The model under review builds one solid part; all positions refer to its coordinate system, in mm. A direction names the side the tool comes from. Coordinates: 2 decimals unless noted, no trailing zeros. Write each loop counter-clockwise with the first axis right and the second up, starting at its lowest first coordinate (ties: lowest second). Pieces come first, ordered by that corner, then holes. Notation, with made-up numbers: (7.5, -7) - (37.5, -7) arc R25 cw to (37.5, 21) - close; hole circle Ø9 at (-25, 58). An arc over 180 degrees is marked (long way). Put each result on its own line as item: value.
from build123d import *

# Parameters (mm, degrees)
SKETCH_W        = 40
SKETCH_H        = 40
SKETCH_R        = 6
SKETCH_R_2      = 1.75
PAD_DEPTH       = 8
SKETCH001_R     = 9.7
POCKET_DEPTH    = 6
SKETCH002_W     = 42
SKETCH002_H     = 42
SKETCH002_R     = 15
POCKET001_DEPTH = 5
FILLET_R        = 3
FILLET001_R     = 3


with BuildPart() as part:
    # Sketch → Pad (new body)
    with BuildSketch(Plane.XY):
        Rectangle(SKETCH_W, SKETCH_H)
        Circle(SKETCH_R, mode=Mode.SUBTRACT)
        with Locations((15.6, 15.6)):
            Circle(SKETCH_R_2, mode=Mode.SUBTRACT)
        with Locations((15.6, -15.6)):
            Circle(SKETCH_R_2, mode=Mode.SUBTRACT)
        with Locations((-15.6, -15.6)):
            Circle(SKETCH_R_2, mode=Mode.SUBTRACT)
        with Locations((-15.6, 15.6)):
            Circle(SKETCH_R_2, mode=Mode.SUBTRACT)
    extrude(amount=PAD_DEPTH)

    # Sketch001 → Pocket (cut)
    with BuildSketch(Plane.XY.offset(8)):
        Circle(SKETCH001_R)
    extrude(amount=-POCKET_DEPTH, mode=Mode.SUBTRACT)

    # Sketch002 → Pocket001 (cut)
    with BuildSketch(Plane.XY.offset(8)):
        Rectangle(SKETCH002_W, SKETCH002_H)
        Circle(SKETCH002_R, mode=Mode.SUBTRACT)
    extrude(amount=-POCKET001_DEPTH, mode=Mode.SUBTRACT)

    # Fillet
    fillet_edges = [part.edges().sort_by_distance(p)[0] for p in [
        (-15, 0, 3),
    ]]
    fillet(fillet_edges, radius=FILLET_R)

    # Fillet001
    fillet001_edges = [part.edges().sort_by_distance(p)[0] for p in [
        (-20, 20, 1.5),
        (20, 20, 1.5),
        (20, -20, 1.5),
        (-20, -20, 1.5),
    ]]
    fillet(fillet001_edges, radius=FILLET001_R)


solid = part.part
1. Consider section D-D on y = 15.6. Give the number of separate pieces and of enclosed holes in the cut face, plus the area to 3 significant figures.
Determined:
separate pieces: 3
enclosed holes: 0
area: 110 mm^2
2. For pin 1 Ø3 at (x, y) = (15.6, -15.6) entering from -Z; pin 2 Ø3 at (x, y) = (16, 8) entering from +Z; pin 3 Ø4 at (x, y) = (-15.6, 15.6) entering from +Z; pin 4 Ø15.5 at (x, y) = (0, 0) entering from +Z, all flat-tipped, find the tip position at first contact; note any pin that passes through.
Determined:
pin 1: passes through
pin 2: stops at z = 3.47
pin 3: stops at z = 3
pin 4: stops at z = 2
3. Machinability: for faces 1 (the cylindrical face through (-14.985, 0.66, 7.014)), 2 (the cylindrical face through (17.217, 14.93, 1.479)), which of the approach directions +Z, -Z, +X, -X, +Y, -Y give a long, thin tool a straight path to every point of the face, cutting with its end or side? Answer none if there is none.
Determined:
face 1: +Z
face 2: +Z, -Z
4. The part is to be moulded in two halves that separate along Y. For faces 3 (the cylindrical face through (15.22, -17.31, 1.48)), 4 (the flat face through (0, -10, 8)), 5 (the flat face through (0, 20, 1)), 6 (the cylindrical face through (-19.14, -19.1, 1.52)), say which applies: +Y half, -Y half, draft (parallel to the pull), parting line (faces both ways), or undercut.
Determined:
face 3: undercut
face 4: draft
face 5: +Y half
face 6: -Y half
5. Consider section B-B on z = 1.25. State the section outline as (x, y) points.
Determined:
outline: (-20, -17) arc R3 ccw to (-17, -20) - (17, -20) arc R3 ccw to (20, -17) - (20, 17) arc R3 ccw to (17, 20) - (-17, 20) arc R3 ccw to (-20, 17) - close; hole circle Ø3.5 at (-15.6, -15.6); hole circle Ø3.5 at (-15.6, 15.6); hole circle Ø12 at (0, 0); hole circle Ø3.5 at (15.6, -15.6); hole circle Ø3.5 at (15.6, 15.6)
6. To check wall thickness, follow probe 1 along Y at (x, z) = (-15.6, 0.8); probe 2 along Y at (x, z) = (0, 1.15); probe 3 along X at (y, z) = (-16.5, 0.75). State the ranges of each line that lie inside material, in increasing order.
Determined:
probe 1: y = -20 to -17.35, -13.85 to 13.85, 17.35 to 20
probe 2: y = -20 to -6, 6 to 20
probe 3: x = -20 to -17.1, -14.1 to 14.1, 17.1 to 20
7. Consider section C-C on z = 7. State the section outline as (x, y) points.
Determined:
outline: circle Ø30 at (0, 0); hole circle Ø19.4 at (0, 0)
8. Consider section A-A on x = 0. State the section outline as (y, z) points, plus the area to 3 significant figures.
Determined:
outline: (-20, 0) - (-6, 0) - (-6, 2) - (-9.7, 2) - (-9.7, 8) - (-15, 8) - (-15, 6) arc R3 cw to (-18, 3) - (-20, 3) - close; (6, 0) - (20, 0) - (20, 3) - (18, 3) arc R3 cw to (15, 6) - (15, 8) - (9.7, 8) - (9.7, 2) - (6, 2) - close
area: 133 mm^2
